```python
from build123d import *

# Parameters (mm, degrees)
ESQUISSE1_R             = 2.5
BOSS_EXTRU_1_DEPTH      = 3
ENL_V_MAT_EXTRU_1_DEPTH = 166.064843505
SKETCH1_W               = 235.08624341
SKETCH1_H               = 3
BOSS_EXTRUDE1_DEPTH     = 20
SKETCH2_W               = 54.316544192
SKETCH2_H               = 19.777044638
CUT_EXTRUDE1_DEPTH      = 10
CUT_EXTRUDE2_DEPTH      = 10


with BuildPart() as part:
    # Esquisse1 → Boss.-Extru.1 (new body)
    with BuildSketch(Plane(origin=(0, 0, 0), x_dir=(1, 0, 0), z_dir=(0, 1, 0))):
        Polygon((-161.174292495, 18.77), (-161.174292495, -25.5), (-161.174292495, -35.5), (138.625707505, -35.5), (138.625707505, -10.5), (73.911950915, -10.5), (73.911950915, 28.77), (-161.174292495, 28.77), align=None)
        with Locations(Location((-151.374292495, -19.4325, 0), (0, 0, 270))):
            Circle(ESQUISSE1_R, mode=Mode.SUBTRACT)
        with Locations(Location((-151.374292495, 12.7025, 0), (0, 0, 270))):
            Circle(ESQUISSE1_R, mode=Mode.SUBTRACT)
        with Locations(Location((53.661950915, 10.747499922, 0), (0, 0, 270))):
            Circle(ESQUISSE1_R, mode=Mode.SUBTRACT)
        Polygon((114.261515644, -15.687745544), (114.261515644, -18.634239014), (132.625707505, -18.634239014), (132.625707505, -32.887044638), (114.261515644, -32.887044638), (79.109163313, -32.887044638), (79.109163313, -15.687745544), align=None, mode=Mode.SUBTRACT)
    extrude(amount=BOSS_EXTRU_1_DEPTH)

    # Esquisse2 → Enlèv. mat.-Extru.1 (cut, through all)
    with BuildSketch(Plane.XZ):
        with BuildLine():
            Line((7.640390062, -11.635), (7.640390062, 18.365))
            ThreePointArc((7.640390062, 18.365), (15.140390062, 25.865), (22.640390062, 18.365))
            Line((22.640390062, 18.365), (22.640390062, -11.635))
            ThreePointArc((22.640390062, -11.635), (15.140390062, -19.135), (7.640390062, -11.635))
        make_face()
        with BuildLine():
            Line((-51.13117079, -11.635), (-51.13117079, 18.365))
            ThreePointArc((-51.13117079, 18.365), (-43.63117079, 25.865), (-36.13117079, 18.365))
            Line((-36.13117079, 18.365), (-36.13117079, -11.635))
            ThreePointArc((-36.13117079, -11.635), (-43.63117079, -19.135), (-51.13117079, -11.635))
        make_face()
        with BuildLine():
            Line((-109.902731643, -11.635), (-109.902731643, 18.365))
            ThreePointArc((-109.902731643, 18.365), (-102.402731643, 25.865), (-94.902731643, 18.365))
            Line((-94.902731643, 18.365), (-94.902731643, -11.635))
            ThreePointArc((-94.902731643, -11.635), (-102.402731643, -19.135), (-109.902731643, -11.635))
        make_face()
    extrude(amount=-ENL_V_MAT_EXTRU_1_DEPTH, mode=Mode.SUBTRACT)

    # Sketch1 → Boss-Extrude1 (add)
    with BuildSketch(Plane(origin=(0, 0, -28.77), x_dir=(-1, 0, 0), z_dir=(0, 0, -1))):
        with Locations((43.63117079, 1.5)):
            Rectangle(SKETCH1_W, SKETCH1_H)
    extrude(amount=BOSS_EXTRUDE1_DEPTH)

    # Sketch2 → Cut-Extrude1 (cut)
    with BuildSketch(Plane.XZ):
        with Locations((106.267435409, 22.998522319)):
            Rectangle(SKETCH2_W, SKETCH2_H)
    extrude(amount=-CUT_EXTRUDE1_DEPTH, mode=Mode.SUBTRACT)

    # Sketch3 → Cut-Extrude2 (cut)
    with BuildSketch(Plane(origin=(0, 0, 0), x_dir=(-1, 0, 0), z_dir=(0, -1, 0))):
        with BuildLine():
            Line((90.402731643, -18.365), (90.402731643, 31.635))
            ThreePointArc((90.402731643, 31.635), (102.402731643, 43.635), (114.402731643, 31.635))
            Line((114.402731643, 31.635), (114.402731643, -18.365))
            ThreePointArc((114.402731643, -18.365), (102.402731643, -30.365), (90.402731643, -18.365))
        make_face()
        with BuildLine():
            Line((30.402731643, -18.365), (30.402731643, 31.635))
            ThreePointArc((30.402731643, 31.635), (42.402731643, 43.635), (54.402731643, 31.635))
            Line((54.402731643, 31.635), (54.402731643, -18.365))
            ThreePointArc((54.402731643, -18.365), (42.402731643, -30.365), (30.402731643, -18.365))
        make_face()
        with BuildLine():
            Line((-29.597268357, -18.365), (-29.597268357, 31.635))
            ThreePointArc((-29.597268357, 31.635), (-17.597268357, 43.635), (-5.597268357, 31.635))
            Line((-5.597268357, 31.635), (-5.597268357, -18.365))
            ThreePointArc((-5.597268357, -18.365), (-17.597268357, -30.365), (-29.597268357, -18.365))
        make_face()
    extrude(amount=-CUT_EXTRUDE2_DEPTH, mode=Mode.SUBTRACT)


solid = part.part
```
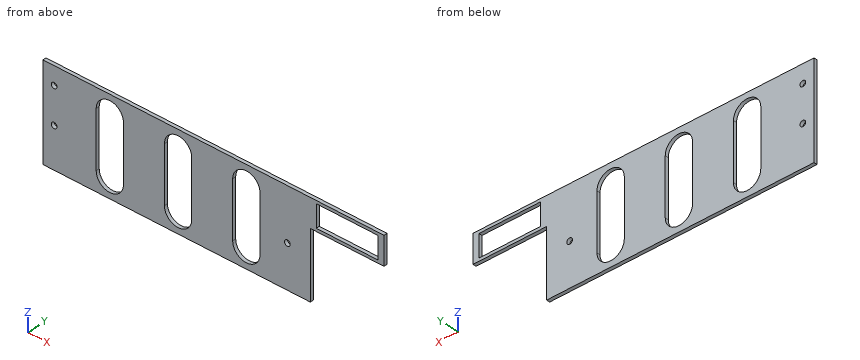
Here's how the part is built. I have some questions about the finished solid (model axes, mm). Coordinates: 2 decimals unless noted, no trailing zeros. Write each loop counter-clockwise with the first axis right and the second up, starting at its lowest first coordinate (ties: lowest second). Pieces come first, ordered by that corner, then holes. Notation, with made-up numbers: (74.5, -18) -> (131.5, -18) arc R24 cw to (131.5, 1) -> close; hole circle Ø2 at (44.25, 66). An arc over 180 degrees is marked (long way). Use a Markdown table: item, result. Add a question column.
(1) I'm going to push flat-ended pins straight in: P1, Ø0.9, axis at y = 1, z = 5, coming from the +X side; P2, Ø0.9, axis at x = 102, y = 1.5, coming from the -Z side; P3, Ø4.5, axis at x = -151.37, z = 19.43, coming from the +Y side. Where does each tip first touch, or does it pass through?
(2) If we section it at D-D, the plane z = -36: Write out the boundary of the cut face in (x, y), and give its area (3 significant figures).
(3) If we section it at A-A, the plane z = 7: Write out the boundary of the cut face in (x, y).
(4) If we section it at C-C, the plane y = 2.2: Write out the boundary of the cut face in (x, z) (1 decimal).
(5) Please list where these lines run through material, in increasing order: line 1 (X direction, y = 0.8, z = 16); line 2 (X direction, y = 1.4, z = -28.5); line 3 (X direction, y = 0.5, z = -8.5).
(6) If we section it at B-B, the plane x = -103: Write out the boundary of the cut face in (y, z).
Outcome:
| question | item | result |
|---|---|---|
| 1 | P1 | stops at x = 73.91 |
| 1 | P2 | stops at z = 10.5 |
| 1 | P3 | passes through |
| 2 | outline | (-161.17, 0) -> (-113.58, 0) -> (-113.58, 3) -> (-161.17, 3) -> close; (-91.22, 0) -> (-53.58, 0) -> (-53.58, 3) -> (-91.22, 3) -> close; (-31.22, 0) -> (6.42, 0) -> (6.42, 3) -> (-31.22, 3) -> close; (28.78, 0) -> (73.91, 0) -> (73.91, 3) -> (28.78, 3) -> close |
| 2 | area | 504 mm^2 |
| 3 | outline | (-161.17, 0) -> (-114.4, 0) -> (-114.4, 3) -> (-161.17, 3) -> close; (-90.4, 0) -> (-54.4, 0) -> (-54.4, 3) -> (-90.4, 3) -> close; (-30.4, 0) -> (5.6, 0) -> (5.6, 3) -> (-30.4, 3) -> close; (29.6, 0) -> (73.91, 0) -> (73.91, 3) -> (29.6, 3) -> close |
| 4 | outline | (-161.2, -48.8) -> (73.9, -48.8) -> (73.9, 10.5) -> (138.6, 10.5) -> (138.6, 35.5) -> (-161.2, 35.5) -> close; hole circle Ø5 at (-151.4, -12.7); hole circle Ø5 at (-151.4, 19.4); hole (-114.4, -31.6) arc R12 ccw to (-90.4, -31.6) -> (-90.4, 18.4) arc R12 ccw to (-114.4, 18.4) -> close; hole (-54.4, -31.6) arc R12 ccw to (-30.4, -31.6) -> (-30.4, 18.4) arc R12 ccw to (-54.4, 18.4) -> close; hole (5.6, -31.6) arc R12 ccw to (29.6, -31.6) -> (29.6, 18.4) arc R12 ccw to (5.6, 18.4) -> close; hole circle Ø5 at (53.7, -10.7); hole (79.1, 13.1) -> (133.4, 13.1) -> (133.4, 32.9) -> (79.1, 32.9) -> close |
| 5 | line 1 | x = -161.17 to -114.4, -90.4 to -54.4, -30.4 to 5.6, 29.6 to 79.11, 133.43 to 138.63 |
| 5 | line 2 | x = -161.17 to -114.4, -90.4 to -54.4, -30.4 to 5.6, 29.6 to 73.91 |
| 5 | line 3 | x = -161.17 to -114.4, -90.4 to -54.4, -30.4 to 5.6, 29.6 to 52.57, 54.76 to 73.91 |
| 6 | outline | (0, -48.77) -> (3, -48.77) -> (3, -43.62) -> (0, -43.62) -> close; (0, 30.35) -> (3, 30.35) -> (3, 35.5) -> (0, 35.5) -> close |
